from build123d import *

# Parameters (mm, degrees)
BASE_FLANGE1_DEPTH = 18
SKETCH6_R          = 1.5875
SKETCH6_W          = 17
SKETCH6_H          = 10
CUT_EXTRUDE1_DEPTH = 53.430906916
SKETCH7_R          = 1.984375
CUT_EXTRUDE2_DEPTH = 53.430906916
FILLET1_R          = 3


# Sheet-metal steps are written as plain solids
with BuildPart() as part:
    # Sketch1 → Base-Flange1 (new, symmetric)
    with BuildSketch(Plane.XY):
        with BuildLine():
            Line((0, 45), (0, 0.7366))
            ThreePointArc((0, 0.7366), (0.215745145, 0.215745145), (0.7366, 0))
            Line((0.7366, 0), (20, 0))
            Line((20, 0), (20, -0.7366))
            Line((20, -0.7366), (0.7366, -0.7366))
            ThreePointArc((0.7366, -0.7366), (-0.30510971, -0.30510971), (-0.7366, 0.7366))
            Line((-0.7366, 0.7366), (-0.7366, 45))
            Line((-0.7366, 45), (0, 45))
        make_face()
    extrude(amount=BASE_FLANGE1_DEPTH, both=True)

    # Sketch6 → Cut-Extrude1 (cut, through all)
    with BuildSketch(Plane(origin=(0, 0, 0), x_dir=(0, 0, -1), z_dir=(1, 0, 0))):
        with Locations(Location((-12.5, 34.2634, 0), (0, 0, 90))):
            Circle(SKETCH6_R)
        with Locations(Location((12.5, 34.2634, 0), (0, 0, 90))):
            Circle(SKETCH6_R)
        with Locations((0, 34.2634)):
            Rectangle(SKETCH6_W, SKETCH6_H)
    extrude(amount=-CUT_EXTRUDE1_DEPTH, mode=Mode.SUBTRACT)

    # Sketch7 → Cut-Extrude2 (cut, through all)
    with BuildSketch(Plane(origin=(0, 0, 0), x_dir=(1, 0, 0), z_dir=(0, 1, 0))):
        with Locations(Location((10, 8, 0), (0, 0, 270))):
            Circle(SKETCH7_R)
        with Locations(Location((10, -8, 0), (0, 0, 270))):
            Circle(SKETCH7_R)
    extrude(amount=-CUT_EXTRUDE2_DEPTH, mode=Mode.SUBTRACT)

    # Fillet1
    fillet1_edges = [part.edges().sort_by_distance(p)[0] for p in [
        (-0.3683, 45, 18),
        (-0.3683, 45, -18),
    ]]
    fillet(fillet1_edges, radius=FILLET1_R)


solid = part.part
The model under review builds one solid part; all positions refer to its coordinate system, in mm. A direction names the side the tool comes from. Give positions to 0.01 mm unless a question says otherwise; leave off trailing zeros. Order: outer loops, then holes, each group sorted by start corner. A loop starts at its lowest first (then second) coordinate and runs counter-clockwise, first axis right, second up. Notation, with made-up numbers: M -26,27.5 L 4,27.5 A18 ccw 4,50.5 Z; hole C 69.25,-29 d10. An arc over 180 degrees is marked long. Use one line per item in the form item = value. Start each with the question number.
Item 1: Insertion check: pin 1 Ø6 at (x, z) = (7, -2) entering from +Y; pin 2 Ø3.5 at (x, z) = (10, -8) entering from -Y; pin 3 Ø0.6 at (x, z) = (-0.5, -1) entering from -Y; pin 4 Ø3.5 at (y, z) = (34.26, 12.5) entering from +X. Each pin has a flat end and moves straight along its axis. Give the tip position at first contact, or say it passes through.
Item 2: We need section A-A on z = -8. Give the boundary of the cut face in (x, y), plus the area to 3 significant figures.
Item 3: We need section D-D on z = -12.5. Give the boundary of the cut face in (x, y), plus the area to 3 significant figures.
Item 4: To check wall thickness, follow line 1 along X through (y, z) = (14, 4.5); line 2 along X through (y, z) = (-0.2, -8). State the ranges of each line that lie inside material, in increasing order. Write a range as from..to.
Item 5: For faces 1 (the cylindrical face through (-0.36, 44.14, -17.1)), 2 (the flat face through (0, 23, 0)), list the 3-axis set-ups (+Z, -Z, +X, -X, +Y, -Y) from which the entire face can be reached by the end or side of a thin tool; tool diameter is ignored.
Item 6: We need section B-B on y = 38. Give the boundary of the cut face in (x, z).
Item 7: We need section C-C on x = 10. Give the boundary of the cut face in (y, z).
Item 8: The part is to be moulded in two halves that separate along X. For faces 3 (the flat face through (-0.737, 23, 0)), 4 (the cylindrical face through (8.24, -0.36, -7.08)), 5 (the cylindrical face through (8.24, -0.36, 8.92)), 6 (the flat face through (10, 0, 0)), say which applies: pulls with the +X half, pulls with the -X half, needs draft (parallel to the pull), parting line crosses it, or undercut.
Completed:
q1.pin_1 = 0
q1.pin_2 = through
q1.pin_3 = -0.4
q1.pin_4 = 0
q2.outline = M -0.74,0.74 A1.47 ccw 0.74,-0.74 L 8.02,-0.74 L 8.02,0 L 0.74,0 A0.74 cw 0,0.74 L 0,29.26 L -0.74,29.26 Z; M -0.74,39.26 L 0,39.26 L 0,45 L -0.74,45 Z; M 11.98,-0.74 L 20,-0.74 L 20,0 L 11.98,0 Z
q2.area = 37.8 mm²
q3.outline = M -0.74,0.74 A1.47 ccw 0.74,-0.74 L 20,-0.74 L 20,0 L 0.74,0 A0.74 cw 0,0.74 L 0,32.68 L -0.74,32.68 Z; M -0.74,35.85 L 0,35.85 L 0,45 L -0.74,45 Z
q3.area = 45.7 mm²
q4.line_1 = -0.74..0
q4.line_2 = -0.4..8.02, 11.98..20
q5.face_1 = -Z, +X, -X, +Y
q5.face_2 = +Z, -Z, +X, +Y
q6.outline = M -0.74,-18 L 0,-18 L 0,-8.5 L -0.74,-8.5 Z; M -0.74,8.5 L 0,8.5 L 0,18 L -0.74,18 Z
q7.outline = M -0.74,-18 L 0,-18 L 0,-9.98 L -0.74,-9.98 Z; M -0.74,-6.02 L 0,-6.02 L 0,6.02 L -0.74,6.02 Z; M -0.74,9.98 L 0,9.98 L 0,18 L -0.74,18 Z
q8.face_3 = pulls with the -X half
q8.face_4 = undercut
q8.face_5 = undercut
q8.face_6 = needs draft
